Here's the drawing with two shaded views (mm, measured from the low corner). I have some questions. A direction names the side the tool comes from. Coordinates: 2 decimals unless noted, no trailing zeros. Order: outer loops, then holes, each group sorted by start corner. A loop starts at its lowest first (then second) coordinate and runs counter-clockwise, first axis right, second up. Notation, with made-up numbers: (-18, 42) - (8, 42) arc R11 cw to (8, 50) - close; hole circle Ø7 at (7.5, 59). An arc over 180 degrees is marked (long way). Answer as a JSON object with one key per item and string values. Group by question number.
(1) Imagine slicing it at A-A, the plane x = 6.35. Give the number of separate pieces and of enclosed holes in the cut face, and give its area (3 significant figures).
(2) Will these pins go through, and if not, where does the flat tip stop? P1, Ø0.9, axis at y = 7, z = 1, coming from the +X side; P2, Ø1.5, axis at x = 14.5, z = 2, coming from the -Y side.
(3) We'd pull the mould along Y, two halves only. Please class the marked faces 4, 5, 6 and 7: pulls with the +Y half, pulls with the -Y half, needs draft (parallel to the pull), parting line crosses it, or undercut.
(4) Imagine slicing it at C-C, the plane y = 58.5. Write out the boundary of the cut face in (x, z).
(5) Please list where these lines run through material, in increasing order: probe 1 along Y at (x, z) = (14.25, 1.95); probe 2 along Y at (x, z) = (14, 1.75); probe 3 along Y at (x, z) = (17, 0.35).
(6) Which directions (+Z, -Z, +X, -X, +Y, -Y) give clear straight access to the entire face, cutting with the end or side of a thin tool? Please do the marked faces 1, 2 and 3.
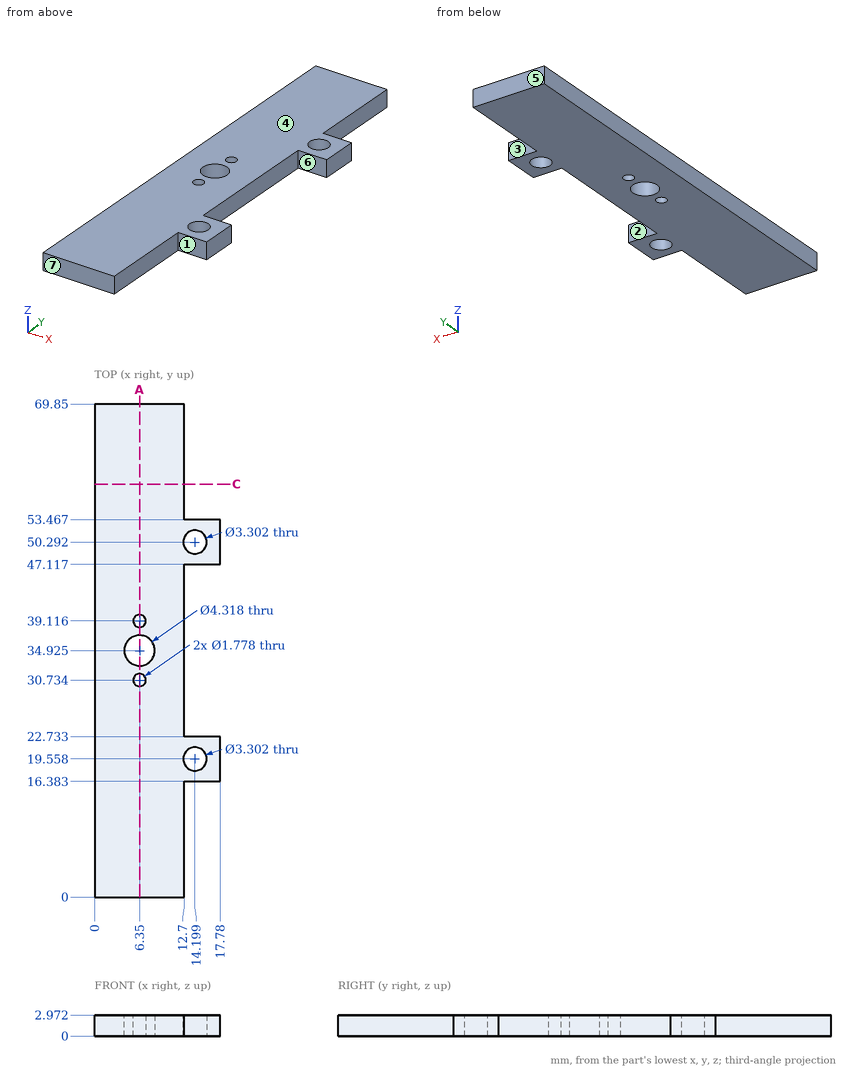
Result set:
{
 "1": {"separate pieces": "4", "enclosed holes": "0", "area": "184 mm^2"},
 "2": {"P1": "stops at x = 12.7", "P2": "stops at y = 16.38"},
 "3": {"face 4": "needs draft", "face 5": "pulls with the +Y half", "face 6": "undercut", "face 7": "pulls with the -Y half"},
 "4": {"outline": "(0, 0) - (12.7, 0) - (12.7, 2.97) - (0, 2.97) - close"},
 "5": {"probe 1": "y = 16.38 to 17.91, 21.21 to 22.73, 47.12 to 48.64, 51.94 to 53.47", "probe 2": "y = 16.38 to 17.92, 21.2 to 22.73, 47.12 to 48.65, 51.93 to 53.47", "probe 3": "y = 16.38 to 22.73, 47.12 to 53.47"},
 "6": {"face 1": "+Z, -Z, +X, -Y", "face 2": "+Z, -Z, +X", "face 3": "+Z, -Z, +X, +Y"}
}
